Could you check a few things on this model? Use its own coordinates, in mm. Round coordinates to 2 decimals unless told otherwise and drop trailing zeros. Loops run counter-clockwise (first coordinate to the right, second up) from the corner with the lowest first, then second, coordinate; pieces in that order, holes last. Notation, with made-up numbers: (51.5, -26) -> (104.5, -26) arc R36 cw to (104.5, 10) -> close; hole circle Ø9 at (56, 40.25). An arc over 180 degrees is marked (long way). One line per item, written item: value.
```python
from build123d import *

# Parameters (mm, degrees)
F0_R     = 13.748153
F0_R_2   = 7.9375
F1_DEPTH = 14
F3_R     = 2.5
F2_R     = 16.813718
F4_DEPTH = 25
F5_SIZE  = 0.5


with BuildPart() as f1:
    # F0 (on Top) → F1 (new body)
    with BuildSketch(Plane.XY):
        Circle(F0_R)
        Circle(F0_R_2, mode=Mode.SUBTRACT)
    extrude(amount=F1_DEPTH)

    # F3
    f3_edges = [f1.edges().sort_by_distance(p)[0] for p in [
        (-13.748153, 0, 14),
        (-13.748153, 0, 0),
    ]]
    fillet(f3_edges, radius=F3_R)

    # F2 (on face) → F4 (cut)
    with BuildSketch(Plane.XY.offset(14)):
        Circle(F2_R)
        Polygon((-11.90625, 6.874077), (0, 13.748153), (11.90625, 6.874077), (11.90625, -6.874077), (0, -13.748153), (-11.90625, -6.874077), align=None, mode=Mode.SUBTRACT)
    extrude(amount=-F4_DEPTH, mode=Mode.SUBTRACT)

    # F5
    f5_edges = [f1.edges().sort_by_distance(p)[0] for p in [
        (7.9375, 0, 7),
        (-7.9375, 0, 0),
        (-7.9375, 0, 14),
    ]]
    chamfer(f5_edges, length=F5_SIZE)


solid = f1.part
```
(1) Imagine slicing it at B-B on z = 9.5. Write out the boundary of the cut face in (x, y) (1 decimal), then the cut area to 3 significant figures.
Results below:
outline: (-11.9, -6.9) -> (0, -13.7) -> (11.9, -6.9) -> (11.9, 6.9) -> (0, 13.7) -> (-11.9, 6.9) -> close; hole circle Ø15.9 at (0, 0)
area: 293 mm²
(2) Imagine slicing it at A-A on y = 0. Write out the boundary of the cut face in (x, z), then the cut area to 3 significant figures.
Results below:
outline: (-11.91, 0.09) arc R2.5 ccw to (-11.25, 0) -> (-8.44, 0) -> (-7.94, 0.5) -> (-7.94, 13.5) -> (-8.44, 14) -> (-11.25, 14) arc R2.5 ccw to (-11.91, 13.91) -> close; (7.94, 0.5) -> (8.44, 0) -> (11.25, 0) arc R2.5 ccw to (11.91, 0.09) -> (11.91, 13.91) arc R2.5 ccw to (11.25, 14) -> (8.44, 14) -> (7.94, 13.5) -> close
area: 111 mm²
(3) Imagine slicing it at C-C on z = 12.5. Write out the boundary of the cut face in (x, y) (1 decimal).
Results below:
outline: (-11.9, -6.4) arc R13.5 ccw to (-11.5, -7.1) -> (-0.4, -13.5) arc R13.5 ccw to (0.4, -13.5) -> (11.5, -7.1) arc R13.5 ccw to (11.9, -6.4) -> (11.9, 6.4) arc R13.5 ccw to (11.5, 7.1) -> (0.4, 13.5) arc R13.5 ccw to (-0.4, 13.5) -> (-11.5, 7.1) arc R13.5 ccw to (-11.9, 6.4) -> close; hole circle Ø15.9 at (0, 0)
(4) Please list where these lines run through material, in increasing order: L1, parallel to Y at x = -2, z = 11; L2, parallel to Y at x = 5.75, z = 10.25; L3, parallel to X at y = 4, z = 11.25.
Results below:
L1: y = -12.59 to -7.68, 7.68 to 12.59
L2: y = -10.43 to -5.47, 5.47 to 10.43
L3: x = -11.91 to -6.86, 6.86 to 11.91
(5) For pin 1 Ø6 at (x, z) = (4, 7.5) entering from +Y; pin 2 Ø2 at (y, z) = (11, 8) entering from +X; pin 3 Ø8 at (x, z) = (-9, 9.5) entering from +Y, each with a flat end and sliding along its axis, tell me the tip position at first contact or that it passes through.
Results below:
pin 1: stops at y = 13.17
pin 2: stops at x = 6.49
pin 3: stops at y = 10.86
(6) We'd pull the mould along Y, two halves only. Please class faces 1 (the face through (-1.72, -7.75, 6.91)), 2 (the face through (5.87, 10.36, 7.1)), 3 (the face through (4, 8, 0)): +Y half, -Y half, draft (parallel to the pull), parting line (faces both ways), or undercut.
Results below:
face 1: undercut
face 2: +Y half
face 3: draft
